Could you check a few things on this model? Use its own coordinates, in mm. Round coordinates to 2 decimals unless told otherwise and drop trailing zeros. One line per item, written item: value.
from build123d import *

# Parameters (mm, degrees)
BOSS_EXTRUDE1_DEPTH   = 6
F_4_0MM_DOWEL_HOLE1_D = 4
F_4_0MM_DOWEL_HOLE2_D = 4


with BuildPart() as part:
    # Sketch1 → Boss-Extrude1 (new body)
    with BuildSketch(Plane(origin=(0, 0, 0), x_dir=(1, 0, 0), z_dir=(0, 1, 0))):
        with BuildLine():
            Line((2499.703486599, -171.073776325), (2596, -162.925319615))
            Line((2596, -162.925319615), (2596, -65.415893177))
            Line((2596, -65.415893177), (2424.991970984, -63.971373722))
            ThreePointArc((2424.991970984, -63.971373722), (2402.577804859, -116.816939936), (2349.361137771, -138.3351893))
            Line((2349.361137771, -138.3351893), (2049.371840186, -135.801154032))
            ThreePointArc((2049.371840186, -135.801154032), (1996.526273972, -113.386987906), (1975.008024607, -60.170320818))
            Line((1975.008024607, -60.170320818), (1824.991970984, -58.903122375))
            ThreePointArc((1824.991970984, -58.903122375), (1802.577804859, -111.74868859), (1749.361137771, -133.266937954))
            Line((1749.361137771, -133.266937954), (1449.371840186, -130.732902685))
            ThreePointArc((1449.371840186, -130.732902685), (1396.526273972, -108.31873656), (1375.008024607, -55.102069472))
            Line((1375.008024607, -55.102069472), (1224.991970984, -53.834871029))
            ThreePointArc((1224.991970984, -53.834871029), (1202.577804859, -106.680437244), (1149.361137771, -128.198686608))
            Line((1149.361137771, -128.198686608), (849.371840186, -125.664651339))
            ThreePointArc((849.371840186, -125.664651339), (796.526273972, -103.250485214), (775.008024607, -50.033818126))
            Line((775.008024607, -50.033818126), (603.999995592, -48.58929867))
            Line((603.999995592, -48.58929867), (603.999995592, -178.649131079))
            Line((603.999995592, -178.649131079), (700.169555672, -189.82522818))
            Line((700.169555672, -189.82522818), (699.325355788, -197.780561394))
            add(Edge.make_bspline(
                [(1279.993726967, -230.586145743), (1251.992845438, -230.214377978), (1156.643871099, -228.426153503), (993.973907449, -222.123757287), (828.430766092, -210.545808412), (730.308385941, -201.068402366), (699.325355788, -197.780561394)],
                knots=[0.338165656, 0.338165656, 0.338165656, 0.338165656, 0.348560819, 0.373566506, 0.398590699, 0.410156143, 0.410156143, 0.410156143, 0.410156143], degree=3))
            Line((1279.993726967, -230.586145743), (1280.033554464, -227.586410126))
            Line((1280.033554464, -227.586410126), (1299.031880037, -227.838650935))
            Line((1299.031880037, -227.838650935), (1299.496534159, -192.841735406))
            Line((1299.496534159, -192.841735406), (1301.496357904, -192.86828707))
            Line((1301.496357904, -192.86828707), (1301.031703781, -227.865202599))
            Line((1301.031703781, -227.865202599), (1320.030029354, -228.117443409))
            Line((1320.030029354, -228.117443409), (1320.006426802, -231.014189882))
            add(Edge.make_bspline(
                [(1880.017536915, -218.975094986), (1786.718289466, -223.252626978), (1600.105449253, -230.003314719), (1413.337833656, -231.774649729), (1320.006426802, -231.014189882)],
                knots=[0.263896993, 0.263896993, 0.263896993, 0.263896993, 0.298568064, 0.333214348, 0.333214348, 0.333214348, 0.333214348], degree=3))
            Line((1880.017536915, -218.975094986), (1879.880138913, -215.978243006))
            Line((1879.880138913, -215.978243006), (1898.859006014, -215.082361576))
            Line((1898.859006014, -215.082361576), (1897.208698115, -180.121290599))
            Line((1897.208698115, -180.121290599), (1899.2064736, -180.02698729))
            Line((1899.2064736, -180.02698729), (1900.856781499, -214.988058267))
            Line((1900.856781499, -214.988058267), (1919.8356486, -214.092176836))
            Line((1919.8356486, -214.092176836), (1919.981085174, -217.088649463))
            add(Edge.make_bspline(
                [(2500.358506516, -179.046915538), (2467.819448595, -181.720107419), (2301.688178219, -194.916310103), (2108.203569807, -207.523423052), (1947.177539067, -215.76864439), (1919.981085174, -217.088649463)],
                knots=[0.186972113, 0.186972113, 0.186972113, 0.186972113, 0.199092181, 0.248838609, 0.258946381, 0.258946381, 0.258946381, 0.258946381], degree=3))
            Line((2500.358506516, -179.046915538), (2499.703486599, -171.073776325))
        make_face()
        with BuildLine():
            Line((2499.792273349, 35.207087267), (2500.052462016, 43.202855013))
            add(Edge.make_bspline(
                [(1919.991369728, 61.760722375), (1946.141292077, 60.986188213), (2105.246296635, 56.201656656), (2298.592719455, 49.780680894), (2465.794842369, 44.317625311), (2500.052462016, 43.202855013)],
                knots=[0.742494138, 0.742494138, 0.742494138, 0.742494138, 0.752206114, 0.801585908, 0.814310206, 0.814310206, 0.814310206, 0.814310206], degree=3))
            Line((1919.991369728, 61.760722375), (1919.903226355, 58.762017531))
            Line((1919.903226355, 58.762017531), (1900.911429005, 59.320258891))
            Line((1900.911429005, 59.320258891), (1899.883089657, 24.335369036))
            Line((1899.883089657, 24.335369036), (1897.883953094, 24.394131284))
            Line((1897.883953094, 24.394131284), (1898.912292442, 59.379021139))
            Line((1898.912292442, 59.379021139), (1879.920499189, 59.93726238))
            Line((1879.920499189, 59.93726238), (1880.008642561, 62.935967224))
            add(Edge.make_bspline(
                [(1319.993980998, 78.100288692), (1413.331517369, 75.731088455), (1600.006544772, 70.824745257), (1786.675707055, 65.658872993), (1880.008642561, 62.935967224)],
                knots=[0.668220223, 0.668220223, 0.668220223, 0.668220223, 0.70288135, 0.737544363, 0.737544363, 0.737544363, 0.737544363], degree=3))
            Line((1319.993980998, 78.100288692), (1319.917856082, 75.101254681))
            Line((1319.917856082, 75.101254681), (1300.923911605, 75.580914146))
            Line((1300.923911605, 75.580914146), (1300.040328379, 40.592069057))
            Line((1300.040328379, 40.592069057), (1298.040965803, 40.642559527))
            Line((1298.040965803, 40.642559527), (1298.924549029, 75.631404616))
            Line((1298.924549029, 75.631404616), (1279.930604552, 76.111064082))
            Line((1279.930604552, 76.111064082), (1280.005946886, 79.110117855))
            add(Edge.make_bspline(
                [(699.999889789, 89.613058052), (735.879488596, 89.493405625), (837.870012607, 88.671897295), (1005.865228965, 85.782705717), (1163.311518707, 82.018687941), (1254.670838845, 79.746587332), (1280.005946886, 79.110117855)],
                knots=[0.591485773, 0.591485773, 0.591485773, 0.591485773, 0.604805069, 0.629344389, 0.653862178, 0.663270358, 0.663270358, 0.663270358, 0.663270358], degree=3))
            Line((699.999889789, 89.613058052), (699.973211283, 81.613102536))
            Line((699.973211283, 81.613102536), (603.999995592, 81.470533738))
            Line((603.999995592, 81.470533738), (603.999995592, -48.58929867))
            Line((603.999995592, -48.58929867), (775.008024607, -50.033818126))
            ThreePointArc((775.008024607, -50.033818126), (797.422190733, 2.811748089), (850.638857821, 24.329997453))
            Line((850.638857821, 24.329997453), (1150.628155405, 21.795962184))
            ThreePointArc((1150.628155405, 21.795962184), (1203.47372162, -0.618203941), (1224.991970984, -53.834871029))
            Line((1224.991970984, -53.834871029), (1375.008024607, -55.102069472))
            ThreePointArc((1375.008024607, -55.102069472), (1397.422190733, -2.256503257), (1450.638857821, 19.261746107))
            Line((1450.638857821, 19.261746107), (1750.628155405, 16.727710838))
            ThreePointArc((1750.628155405, 16.727710838), (1803.47372162, -5.686455287), (1824.991970984, -58.903122375))
            Line((1824.991970984, -58.903122375), (1975.008024607, -60.170320818))
            ThreePointArc((1975.008024607, -60.170320818), (1997.422190733, -7.324754603), (2050.638857821, 14.193494761))
            Line((2050.638857821, 14.193494761), (2350.628155405, 11.659459492))
            ThreePointArc((2350.628155405, 11.659459492), (2403.47372162, -10.754706634), (2424.991970984, -63.971373722))
            Line((2424.991970984, -63.971373722), (2596, -65.415893177))
            Line((2596, -65.415893177), (2596, 32.093533261))
            Line((2596, 32.093533261), (2499.792273349, 35.207087267))
        make_face()
    extrude(amount=BOSS_EXTRUDE1_DEPTH)

    # Ø4.0mm Dowel Hole1 (through all)
    with Locations(Plane(origin=(2535.820689775, 0, 65.575730663), x_dir=(0, 0, -1), z_dir=(0, -1, 0))):
        with Locations((0, 0), (-40, 0), (-80, 0), (40, 0), (80, 0)):
            Hole(F_4_0MM_DOWEL_HOLE1_D / 2)

    # Ø4.0mm Dowel Hole2 (through all)
    with Locations(Plane(origin=(664.175101974, 0, 48.706016617), x_dir=(0, 0, -1), z_dir=(0, -1, 0))):
        with Locations((0, 0), (-80, 0), (-40, 0), (80, 0), (40, 0)):
            Hole(F_4_0MM_DOWEL_HOLE2_D / 2)


solid = part.part
(1) If I drill on L1, parallel to X at y = 1.25, z = 93.5; L2, parallel to X at y = 0.5, z = -3; L3, parallel to Z at x = 1464, y = 5.25, over which ranges is the centre line in solid material (lowest first)?
Recorded:
L1: 604 to 788.44, 1213.25 to 1385.21, 1816.21 to 1982.51, 2418.66 to 2596
L2: 604 to 797.61, 1199.66 to 1403.37, 1793.25 to 2010.58, 2384.98 to 2596
L3: -74.38 to -19.15, 130.86 to 230.94
(2) If we section it at A-A, the plane y = 1: Give the number of separate pieces and of enclosed holes in the cut face, then the cut area to 3 significant figures.
Recorded:
separate pieces: 1
enclosed holes: 13
area: 369,000 mm²
(3) Thinking about a two-plate mould opening in X: for faces 1 (the face through (1586, 6, 140)), 2 (the face through (2424.988, 2.958, 62.322)), which applies, released by +X, released by -X, zero draft, split by the parting line, or undercut?
Recorded:
face 1: zero draft
face 2: undercut
